Here's how the part is built. I have some questions about the finished solid (model axes, mm). A direction names the side the tool comes from. Give positions to 0.01 mm unless a question says otherwise; leave off trailing zeros. Write each loop counter-clockwise with the first axis right and the second up, starting at its lowest first coordinate (ties: lowest second). Pieces come first, ordered by that corner, then holes. Notation, with made-up numbers: (-20, 46.25) -> (-14, 46.25) arc R29 ccw to (-14, 76.25) -> close; hole circle Ø1 at (48.25, 16). An arc over 180 degrees is marked (long way). Use CSV: the item, a comma, the result in double quotes. Start each with the question number.
(1) Suppose I cut it at C-C on y = 125. List the corners of the cut face in (x, z) for me.
(2) For pin 1 Ø1 at (x, y) = (43, 30.5) entering from -Z; pin 2 Ø1.5 at (y, z) = (41.5, -46.5) entering from +X, each with a flat end and sliding along its axis, tell me the tip position at first contact or that it passes through.
(3) Suppose I cut it at B-B on y = 25. List the corners of the cut face in (x, z) for me.
(4) Suppose I cut it at A-A on x = 37.5. List the corners of the cut face in (y, z) for me, plus the area to 3 significant figures.
(5) Which directions (+Z, -Z, +X, -X, +Y, -Y) give clear straight access to the entire face, cutting with the end or side of a thin tool? Please do faces 1 (the flat face through (2, 59, -65)), 2 (the flat face through (4, 69, -34)).
(6) Suppose I cut it at D-D on z = -9. List the corners of the cut face in (x, y) for me, plus the area to 3 significant figures.
(7) I need wall thicknesses on L1, parallel to Y at x = 37, z = -1; L2, parallel to X at y = 75, z = -1.9; L3, parallel to Z at x = 11.5, y = 169.5. Which ranges of each line are inside material? Lowest first, please. Write a range as [from, to].
(8) If we mould it in two halves opening along X, with no side actions, what happens to faces 3 (the cylindrical face through (41.5, 22, -2)), 4 (the flat face through (65, 89, -2)), 5 (the flat face through (2, 149, -35))? For each: pulls with the +X half, pulls with the -X half, needs draft (parallel to the pull), parting line crosses it, or undercut.
from build123d import *

# Parameters (mm, degrees)
EXTRUDE_1_DEPTH     = 180
SKETCH_6_R          = 5
CUT_EXTRUDE_1_DEPTH = 10
CUT_EXTRUDE_2_DEPTH = 10


with BuildPart() as part:
    # Эскиз1 → Вытянуть-Тонкостенный1 (new body)
    with BuildSketch(Plane(origin=(0, 0, 0), x_dir=(1, 0, 0), z_dir=(0, 1, 0))):
        Polygon((0, 65), (0, 0), (65, 0), (65, 4), (4, 4), (4, 65), align=None)
    extrude(amount=EXTRUDE_1_DEPTH)

    # Эскиз6 → Вырез-Вытянуть1 (cut)
    with BuildSketch(Plane(origin=(0, 0, 0), x_dir=(-1, 0, 0), z_dir=(0, 0, -1))):
        with Locations((-37.5, 25)):
            Circle(SKETCH_6_R)
        with Locations((-37.5, 75)):
            Circle(SKETCH_6_R)
        with Locations((-37.5, 125)):
            Circle(SKETCH_6_R)
    extrude(amount=CUT_EXTRUDE_1_DEPTH, mode=Mode.SUBTRACT)

    # Эскиз9 → Вырез-Вытянуть2 (cut)
    with BuildSketch(Plane.ZY):
        Polygon((-4, 180), (-65, 180), (-65, 119), align=None)
    extrude(amount=-CUT_EXTRUDE_2_DEPTH, mode=Mode.SUBTRACT)


solid = part.part
Geometry says:
1,outline,"(0, -59) -> (4, -59) -> (4, -4) -> (32.5, -4) -> (32.5, 0) -> (0, 0) -> close; (42.5, -4) -> (65, -4) -> (65, 0) -> (42.5, 0) -> close"
2,pin 1,"z = -4"
2,pin 2,"x = 4"
3,outline,"(0, -65) -> (4, -65) -> (4, -4) -> (32.5, -4) -> (32.5, 0) -> (0, 0) -> close; (42.5, -4) -> (65, -4) -> (65, 0) -> (42.5, 0) -> close"
4,outline,"(0, -4) -> (20, -4) -> (20, 0) -> (0, 0) -> close; (30, -4) -> (70, -4) -> (70, 0) -> (30, 0) -> close; (80, -4) -> (120, -4) -> (120, 0) -> (80, 0) -> close; (130, -4) -> (180, -4) -> (180, 0) -> (130, 0) -> close"
4,area,"600 mm²"
5,face 1,"-Z, +X, -X, +Y, -Y"
5,face 2,"-Z, +X, +Y, -Y"
6,outline,"(0, 0) -> (4, 0) -> (4, 175) -> (0, 175) -> close"
6,area,"700 mm²"
7,L1,"[0, 20.03], [29.97, 70.03], [79.97, 120.03], [129.97, 180]"
7,L2,"[0, 32.5], [42.5, 65]"
7,L3,"[-4, 0]"
8,face 3,"undercut"
8,face 4,"pulls with the +X half"
8,face 5,"needs draft"
